Can you work these out from the model? Positions are in its coordinate system, mm. Face numbers are marked on the shaded views. A direction names the side the tool comes from. Give positions to 0.01 mm unless a question says otherwise; leave off trailing zeros. Order: outer loops, then holes, each group sorted by start corner. A loop starts at its lowest first (then second) coordinate and runs counter-clockwise, first axis right, second up. Notation, with made-up numbers: M -37,27.25 L 3,27.25 A30 cw 3,66.25 Z; hole C 33.25,63.5 d9. An arc over 180 degrees is marked long. One line per question, with ' | ' between items. Start each with the question number.
1) If we section it at A-A, the plane y = 7.5: State how many separate pieces and enclosed holes the cut face has, plus the area to 3 significant figures.
2) I'm going to push flat-ended pins straight in: pin 1 Ø6 at (y, z) = (-22, 26.5) entering from +X; pin 2 Ø4 at (y, z) = (36.5, 119) entering from -X. Where does each tip first touch, or does it pass through?
3) If we section it at C-C, the plane z = 33: Please give me the cut outline in (x, y) (3 decimals).
4) Please list where these lines run through material, in increasing order: line 1 along X through (y, z) = (0, 41); line 2 along Y through (x, z) = (0, 42.2); line 3 along Z through (x, y) = (42, -6). Write a range as [from, to].
5) Thinking about a two-plate mould opening in Y: for the marked faces 1 and 2, which applies, +Y half, -Y half, draft (parallel to the pull), parting line (faces both ways), or undercut?
6) If we section it at B-B, the plane x = 54.5: Please give me the cut outline in (y, z).
7) For the marked faces 3 and 4, which set-ups out of +Z, -Z, +X, -X, +Y, -Y let a thin tool reach every point of the face, with its end or its side?
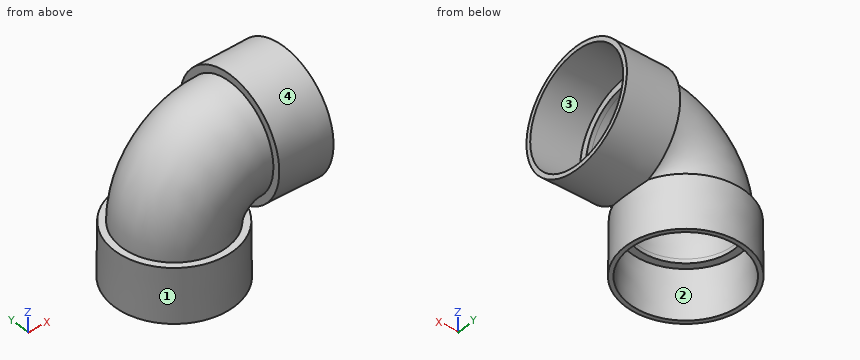
Autodesk Inventor part; units mm, degrees
ref_plane "YZ Plane" through (0, 0, 0) normal (1, 0, 0) x (0, 1, 0)
ref_plane "XZ Plane" through (0, 0, 0) normal (0, 1, 0) x (-1, 0, 0)
ref_plane "XY Plane" through (0, 0, 0) normal (0, 0, 1) x (1, 0, 0)
sketch "Sketch1" plane through (0, 0, 0) normal (0, 1, 0) x (-1, 0, 0)
  line L0 (0, 0) -> (0, 43.4)
  line L1 (48.1252, 0) -> (0, 0)
  line L2 (0, 43.4) -> (47.6912, 43.4)
  line L3 (44.325, 40) -> (44.725, 0)
  line L4 (48.1252, 0) -> (47.6912, 43.4)
  line L5 (38.6, 43.4) -> (38.6, 40)
  line L6 (38.6, 40) -> (44.325, 40)
  line L7 (38.6, 40) -> (0, 40) construction
  dimension "d0" = 89.45
  dimension "d3" = 88.65
  dimension "d4" = 3.4
  dimension "d5" = 40
  dimension "d6" = 3.4
  dimension "d7" = 77.2
revolve "Revolution1" add sketch "Sketch1" angle 360 about axis through (0, 0, 0) along (0, 0, 1) contours L3 L6 L5 L2 L4 L1
sketch "Sketch2" plane through (0, 0, 43.4) normal (0, 0, 1) x (1, 0, 0)
  circle A0 centre (0, 0) radius 47.6912
  circle A1 centre (0, 0) radius 38.6
  circle A2 centre (0, 0) radius 42.2
  circle A3 centre (0, 0) radius 38.6
  dimension "d8" = 77.2
  dimension "d9" = 3.6
sketch "Sketch3" plane through (0, 0, 0) normal (0, 1, 0) x (-1, 0, 0)
  arc A0 (0, 43.4) -> (-44.6, 88) centre (-44.6, 43.4) ccw
  dimension "d10" = 44.6
  dimension "d11" = 44.6
  dimension "d12" = 44.6
sweep "Sweep1" add profiles "Sketch2" path "Sketch3" contours A2
sketch "Sketch4" plane through (0, 0, 0) normal (0, 1, 0) x (-1, 0, 0)
  line L0 (-44.6, 49.4) -> (-44.6, 126.6)
  line L1 (-88, 88) -> (-44.6, 88)
  line L2 (-44.6, 88) -> (-44.6, 135.8912)
  line L3 (-44.6, 135.8912) -> (-88, 136.3252)
  line L4 (-88, 136.3252) -> (-88, 88)
  line L5 (-88, 132.725) -> (-48, 132.325)
  line L6 (-48, 135.9252) -> (-48, 126.6)
  line L7 (-48, 126.6) -> (-44.6, 126.6)
  line L8 (-48, 126.6) -> (-48, 88) construction
  dimension "d14" = 3.6
  dimension "d15" = 40
  dimension "d16" = 3.4
  dimension "d17" = 89.45
  dimension "d18" = 88.65
  dimension "d19" = 77.2
revolve "Revolution2" add sketch "Sketch4" angle 360 about axis through (88, 0, 88) along (-1, 0, 0) contours L7 L6 L3 L2 | L4 L3 L6 L5
equation "\"d0\" = d1"
equation "\"d3\" = d2"
equation "\"d4\" = t2"
equation "\"d5\" = l1"
equation "\"d6\" = t2"
equation "\"d7\" = d"
equation "\"d8\" = d"
equation "\"d9\" = t1"
equation "\"d10\" = Z - t2"
equation "\"d11\" = Z - t2"
equation "\"d12\" = Z - t2"
equation "\"d14\" = t1"
equation "\"d15\" = l1"
equation "\"d16\" = t2"
equation "\"d17\" = d1"
equation "\"d18\" = d2"
equation "\"d19\" = d"
equation "\"d\" = 77.2"
equation "\"d1\" = 89.45"
equation "\"d2\" = 88.65"
equation "\"l1\" = 40"
equation "\"L\" = 88"
equation "\"t1\" = 3.6"
equation "\"t2\" = 3.4"
equation "\"Z\" = 48"
properties part number "JIS K 6739 90 Deg Elbow (DL) 75" material "PVC, Unplasticized"
Results found:
1) separate pieces: 2 | enclosed holes: 1 | area: 1,200 mm²
2) pin 1: stops at x = 43.93 | pin 2: stops at x = 44.6
3) outline: C 0,0 d95.59; hole C 0,0 d88.79
4) line 1: x = [-47.72, -38.6], [38.6, 88] | line 2: y = [-47.7, -38.6], [38.6, 47.7] | line 3: z = [40, 43.4], [44.51, 49.32], [126.09, 129.73]
5) face 1: parting line | face 2: undercut
6) outline: C 0,88 d95.98; hole C 0,88 d88.78
7) face 3: +X | face 4: none
